Build history of the part. All positions in model axes, mm. Round coordinates to 2 decimals unless told otherwise and drop trailing zeros. Loops run counter-clockwise (first coordinate to the right, second up) from the corner with the lowest first, then second, coordinate; pieces in that order, holes last. Notation, with made-up numbers: (80.5, 53) -> (134.5, 53) arc R35 ccw to (134.5, 88) -> close; hole circle Ø8 at (77.5, 55). An arc over 180 degrees is marked (long way). Put each result on its own line as item: value. Start each with the question number.
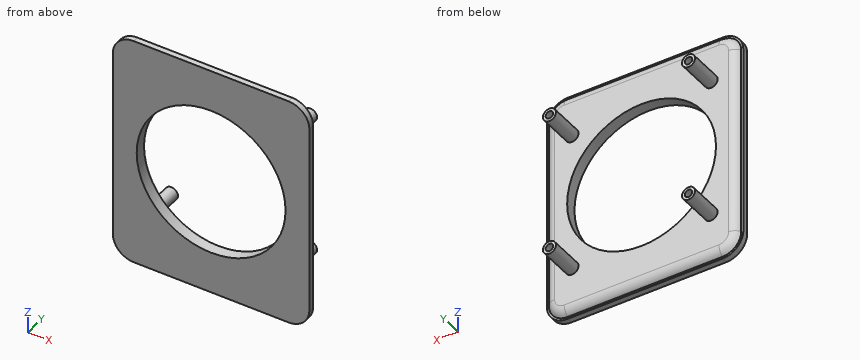
Autodesk Inventor part; units mm, degrees
ref_plane "YZ Plane" through (0, 0, 0) normal (1, 0, 0) x (0, 1, 0)
ref_plane "XZ Plane" through (0, 0, 0) normal (0, 1, 0) x (-1, 0, 0)
ref_plane "XY Plane" through (0, 0, 0) normal (0, 0, 1) x (1, 0, 0)
sketch "Sketch1" plane through (0, 0, 0) normal (0, 1, 0) x (-1, 0, 0)
  circle A0 centre (0, 0) radius 22.6568
  line L0 (0, 35.306) -> (23.5585, 35.306)
  line L1 (29.9085, 28.956) -> (29.9085, -28.956)
  line L2 (23.5585, -35.306) -> (-23.5585, -35.306)
  line L3 (-29.9085, -28.956) -> (-29.9085, 28.956)
  line L4 (-23.5585, 35.306) -> (0, 35.306)
  arc A1 (29.9085, 28.956) -> (23.5585, 35.306) centre (23.5585, 28.956) ccw
  arc A2 (23.5585, -35.306) -> (29.9085, -28.956) centre (23.5585, -28.956) ccw
  arc A3 (-29.9085, -28.956) -> (-23.5585, -35.306) centre (-23.5585, -28.956) ccw
  arc A4 (-23.5585, 35.306) -> (-29.9085, 28.956) centre (-23.5585, 28.956) ccw
  point P0 (29.9085, 35.306)
  point P1 (29.9085, -35.306)
  point P2 (-29.9085, -35.306)
  dimension "d0" = 45.3136
  dimension "d1" = 35.306
  dimension "d2" = 29.9085
  dimension "d3" = 70.612
  dimension "d4" = 59.817
  dimension "d5" = 6.35
extrude "Extrusion1" add sketch "Sketch1" along normal blind 1.778
sketch "Sketch2" plane through (0, 1.778, 0) normal (0, 1, 0) x (1, 0, 0)
  circle A0 centre (0, 0) radius 22.6568
  line L0 (-23.5585, -35.306) -> (23.5585, -35.306)
  line L1 (29.9085, -28.956) -> (29.9085, 28.956)
  line L2 (23.5585, 35.306) -> (-23.5585, 35.306)
  line L3 (-29.9085, 28.956) -> (-29.9085, -28.956)
  line L4 (0, 35.306) -> (0, 34.671)
  line L5 (29.9085, 0) -> (29.2735, 0)
  line L6 (0, -35.306) -> (0, -34.671)
  line L7 (-29.9085, 0) -> (-29.2735, 0)
  line L8 (0, 34.671) -> (-23.5585, 34.671)
  line L9 (-29.2735, 28.956) -> (-29.2735, 0)
  line L10 (0, 34.671) -> (23.5585, 34.671)
  line L11 (29.2735, 28.956) -> (29.2735, 0)
  line L12 (0, -34.671) -> (23.5585, -34.671)
  line L13 (29.2735, -28.956) -> (29.2735, 0)
  line L14 (0, -34.671) -> (-23.5585, -34.671)
  line L15 (-29.2735, -28.956) -> (-29.2735, 0)
  arc A1 (23.5585, -34.671) -> (29.2735, -28.956) centre (23.5585, -28.956) ccw
  arc A2 (29.2735, 28.956) -> (23.5585, 34.671) centre (23.5585, 28.956) ccw
  arc A3 (-23.5585, 34.671) -> (-29.2735, 28.956) centre (-23.5585, 28.956) ccw
  arc A4 (-29.2735, -28.956) -> (-23.5585, -34.671) centre (-23.5585, -28.956) ccw
  circle A5 centre (0, 0) radius 22.6568
  dimension "d8" = 0.635
  dimension "d9" = 0.635
  dimension "d10" = 0.635
  dimension "d11" = 0.635
  dimension "d12" = 5.715
extrude "Extrusion2" add sketch "Sketch2" along normal blind 1.651
fillet "Fillet1" radius 3.175 8 edges at (27.5996, 3.429, -32.9971) (0, 3.429, -34.671) (-27.5996, 3.429, -32.9971) (-29.2735, 3.429, 0) (-27.5996, 3.429, 32.9971) (0, 3.429, 34.671) (27.5996, 3.429, 32.9971) (29.2735, 3.429, 0)
sketch "Sketch3" plane through (0, 3.429, 0) normal (0, 1, 0) x (1, 0, 0)
  circle A0 centre (0, 0) radius 22.6568
  circle A1 centre (0, 0) radius 25.146
  line L0 (-26.2636, 0) -> (-25.5008, 22.4355)
  line L1 (-22.4355, 25.5008) -> (0, 26.2636)
  line L2 (0, 26.2636) -> (22.4355, 25.5008)
  line L3 (25.5008, 22.4355) -> (26.2636, 0)
  line L4 (26.2636, 0) -> (25.5008, -22.4355)
  line L5 (22.4355, -25.5008) -> (0, -26.2636)
  line L6 (0, -26.2636) -> (-22.4355, -25.5008)
  line L7 (-25.5008, -22.4355) -> (-26.2636, 0)
  arc A2 (25.5008, 22.4355) -> (22.4355, 25.5008) centre (22.3276, 22.3276) ccw
  arc A3 (22.4355, -25.5008) -> (25.5008, -22.4355) centre (22.3276, -22.3276) ccw
  arc A4 (-25.5008, -22.4355) -> (-22.4355, -25.5008) centre (-22.3276, -22.3276) ccw
  arc A5 (-22.4355, 25.5008) -> (-25.5008, 22.4355) centre (-22.3276, 22.3276) ccw
  circle A6 centre (-21.1768, 21.1768) radius 1.9812
  circle A7 centre (-21.1768, 21.1768) radius 1.143
  circle A8 centre (21.1768, 21.1768) radius 1.9812
  circle A9 centre (21.1768, 21.1768) radius 1.143
  circle A10 centre (21.1768, -21.1768) radius 1.9812
  circle A11 centre (21.1768, -21.1768) radius 1.143
  circle A12 centre (-21.1768, -21.1768) radius 1.9812
  circle A13 centre (-21.1768, -21.1768) radius 1.143
  point P0 (25.4, 25.4)
  point P1 (-25.4, -25.4)
  point P2 (-25.4, 25.4)
  point P3 (25.4, -25.4)
  dimension "d20" = 50.8
  dimension "d36" = 50.292
  dimension "d39" = 50.8
  dimension "d40" = 50.8
  dimension "d41" = 50.8
  dimension "d46" = 3.175
  dimension "d47" = 3.9624
  dimension "d48" = 2.286
  dimension "d49" = 3.9624
  dimension "d50" = 2.286
  dimension "d51" = 3.9624
  dimension "d52" = 2.286
  dimension "d53" = 3.9624
  dimension "d54" = 2.286
extrude "Extrusion4" add sketch "Sketch3" along normal blind 10.6172 contours A6 | A8 | A10 | A12
properties part number "Speaker Front Plate"
Item 1: Cut at A-A on y = 12.25. Write the cut outline in (x, z), then the cut area to 3 significant figures.
Item 2: Drop flat-ended pins along their axis: pin 1 (1.1 mm diameter, centred on x = 21.5, z = 21, fed in from +Y); pin 2 (3 mm diameter, centred on x = 23, y = 11.5, fed in from +Z); pin 3 (6 mm diameter, centred on x = -15, y = 9.5, fed in from +Z); pin 4 (3 mm diameter, centred on y = 4, z = -21.5, fed in from -X). Give the stop position or say it passes through.
Item 3: Wall check: line 1 (X direction, y = 1.2, z = 0); line 2 (Y direction, x = 19.5, z = -29); line 3 (Z direction, x = 22, y = 8.5). Give the ranges that are in metal, low to high. Write a range as from..to.
Ans:
1. outline: circle Ø3.96 at (-21.18, -21.18); circle Ø3.96 at (-21.18, 21.18); circle Ø3.96 at (21.18, -21.18); circle Ø3.96 at (21.18, 21.18); hole circle Ø2.29 at (-21.18, -21.18); hole circle Ø2.29 at (-21.18, 21.18); hole circle Ø2.29 at (21.18, -21.18); hole circle Ø2.29 at (21.18, 21.18)
1. area: 32.9 mm2
2. pin 1: stops at y = 3.43
2. pin 2: stops at z = 23.13
2. pin 3: passes through
2. pin 4: stops at x = -28.73
3. line 1: x = -29.91..-22.66, 22.66..29.91
3. line 2: y = 0..3.43
3. line 3: z = -22.98..-21.97, -20.38..-19.37, 19.37..20.38, 21.97..22.98
